Here's how the part is built. I have some questions about the finished solid (model axes, mm). Round coordinates to 2 decimals unless told otherwise and drop trailing zeros. Write each loop counter-clockwise with the first axis right and the second up, starting at its lowest first coordinate (ties: lowest second). Pieces come first, ordered by that corner, then holes. Notation, with made-up numbers: (57.25, 55) - (98.25, 55) arc R30 ccw to (98.25, 83) - close; hole circle Ø1 at (49, 4). An arc over 180 degrees is marked (long way). Write item = value, one per line. Start each with the question number.
Item 1: If we section it at B-B (x = 51): Please give me the cut outline in (y, z).
Item 2: If I drill on line 1 along X through (y, z) = (1.3, -106.5); line 2 along Z through (x, y) = (52.5, 0.35), over which ranges is the centre line in solid material (lowest first)? Write a range as [from, to].
Item 3: If we section it at C-C (y = 1.35): Give the number of separate pieces and of enclosed holes in the cut face, and give its area (3 significant figures).
Item 4: If we section it at A-A (z = -90): Please give me the cut outline in (x, y).
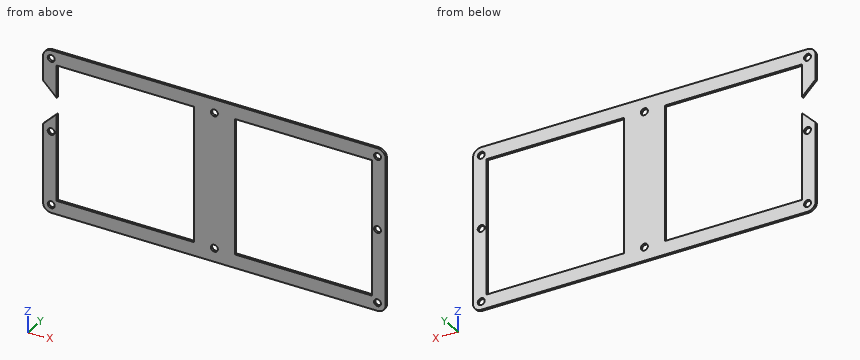
```python
from build123d import *

# Parameters (mm, degrees)
SKETCH_1_R      = 2.55
SKETCH_1_W      = 100
SKETCH_1_H      = 100
EXTRUDE_1_DEPTH = 1.6


with BuildPart() as part:
    # 草图1 → 凸台-拉伸1 (new body)
    with BuildSketch(Plane(origin=(0, 0, 0), x_dir=(1, 0, 0), z_dir=(0, 1, 0))):
        with BuildLine():
            Line((13.495694321, 64.619803607), (13.495694321, 122.619803607))
            ThreePointArc((13.495694321, 122.619803607), (15.253053633, 126.862444294), (19.495694321, 128.619803607))
            Line((19.495694321, 128.619803607), (257.495694321, 128.619803607))
            ThreePointArc((257.495694321, 128.619803607), (261.738335008, 126.862444294), (263.495694321, 122.619803607))
            Line((263.495694321, 122.619803607), (263.495694321, 14.619803607))
            ThreePointArc((263.495694321, 14.619803607), (261.738335008, 10.37716292), (257.495694321, 8.619803607))
            Line((257.495694321, 8.619803607), (19.495694321, 8.619803607))
            ThreePointArc((19.495694321, 8.619803607), (15.253053633, 10.37716292), (13.495694321, 14.619803607))
            Line((13.495694321, 14.619803607), (13.495694321, 32.619803607))
            Line((13.495694321, 32.619803607), (23.495694321, 42.619803607))
            Line((23.495694321, 42.619803607), (23.495694321, 18.619803607))
            Line((23.495694321, 18.619803607), (123.495694321, 18.619803607))
            Line((123.495694321, 18.619803607), (123.495694321, 118.619803607))
            Line((123.495694321, 118.619803607), (23.495694321, 118.619803607))
            Line((23.495694321, 118.619803607), (23.495694321, 54.619803607))
            Line((23.495694321, 54.619803607), (13.495694321, 64.619803607))
        make_face()
        with Locations(Location((19.495694321, 122.619803607, 0), (0, 0, 270))):
            Circle(SKETCH_1_R, mode=Mode.SUBTRACT)
        with Locations(Location((257.495694321, 122.619803607, 0), (0, 0, 270))):
            Circle(SKETCH_1_R, mode=Mode.SUBTRACT)
        with Locations(Location((138.495694321, 118.619803607, 0), (0, 0, 270))):
            Circle(SKETCH_1_R, mode=Mode.SUBTRACT)
        with Locations(Location((19.495694321, 14.619803607, 0), (0, 0, 270))):
            Circle(SKETCH_1_R, mode=Mode.SUBTRACT)
        with Locations(Location((257.495694321, 14.619803607, 0), (0, 0, 270))):
            Circle(SKETCH_1_R, mode=Mode.SUBTRACT)
        with Locations(Location((138.495694321, 18.619803607, 0), (0, 0, 270))):
            Circle(SKETCH_1_R, mode=Mode.SUBTRACT)
        with Locations(Location((257.495694321, 68.619803607, 0), (0, 0, 270))):
            Circle(SKETCH_1_R, mode=Mode.SUBTRACT)
        with Locations(Location((19.495694321, 68.619803607, 0), (0, 0, 270))):
            Circle(SKETCH_1_R, mode=Mode.SUBTRACT)
        with Locations((203.495694321, 68.619803607)):
            Rectangle(SKETCH_1_W, SKETCH_1_H, mode=Mode.SUBTRACT)
    extrude(amount=EXTRUDE_1_DEPTH)


solid = part.part
```
Reply:
q1.outline = (0, -128.62) - (1.6, -128.62) - (1.6, -118.62) - (0, -118.62) - close; (0, -18.62) - (1.6, -18.62) - (1.6, -8.62) - (0, -8.62) - close
q2.line_1 = [13.5, 23.5], [123.5, 153.5], [253.5, 263.5]
q2.line_2 = [-128.62, -118.62], [-18.62, -8.62]
q3.separate_pieces = 1
q3.enclosed_holes = 9
q3.area = 9,590 mm2
q4.outline = (13.5, 0) - (23.5, 0) - (23.5, 1.6) - (13.5, 1.6) - close; (123.5, 0) - (153.5, 0) - (153.5, 1.6) - (123.5, 1.6) - close; (253.5, 0) - (263.5, 0) - (263.5, 1.6) - (253.5, 1.6) - close
